Check sheet for the modelled part. Datum: model origin and axes. Units: mm. A direction names the side the tool comes from. Give positions to 0.01 mm unless a question says otherwise; leave off trailing zeros. Loops run counter-clockwise (first coordinate to the right, second up) from the corner with the lowest first, then second, coordinate; pieces in that order, holes last. Notation, with made-up numbers: (43, -21.75) - (76, -21.75) arc R14 cw to (76, 3.25) - close; hole circle Ø4 at (30, -25.5). An arc over 180 degrees is marked (long way). Answer in a Markdown table with one row per item. Add a question column.
(1) Thickness scan on L1, parallel to X at y = 1.35, z = -80; L2, parallel to X at y = 2.4, z = -32; L3, parallel to Z at x = -32, y = 3.55. Record the ranges inside material, lowest first.
(2) Set-up check for faces 5 (the face through (0, 2, -54)), 6 (the face through (10, 2, -47)): record each of +Z, -Z, +X, -X, +Y, -Y from which the full face is reachable in a straight line by a thin tool's end or side.
(3) Draft check along X on faces 1 (the face through (5.806, 1.972, -81.265)), 2 (the face through (2, 4, -31)), 3 (the face through (-3.01, 2.03, -2.85)), 4 (the face through (8, 2, 9)). Enter one of: released by +X, released by -X, zero draft, split by the parting line, or undercut.
(4) Sectioned sample at C-C on x = -21. Enter the section's corners in (y, z).
(5) Go/stop test with flat-tipped pins: P1, Ø4, axis at x = -31, z = 5, coming from the +Y side; P2, Ø1.5, axis at y = 3, z = -45.5, coming from the -X side; P3, Ø2, axis at x = -20.5, y = 2, coming from the -Z side. Record where each tip stops, or that it passes through.
(6) Sectioned sample at B-B on y = 3.25. Enter the section's corners in (x, z).
(7) Sectioned sample at A-A on x = -31.5. Enter the section's corners in (y, z).
(8) Sectioned sample at D-D on z = -64. Enter the section's corners in (x, y), then the cut area to 3 significant figures.
from build123d import *

# Parameters (mm, degrees)
SKETCH1_R           = 1.5
BOSS_EXTRUDE1_DEPTH = 4
SKETCH2_R           = 2.25
BOSS_EXTRUDE2_DEPTH = 4
FILLET1_R           = 10
FILLET2_R           = 5


with BuildPart() as part:
    # Sketch1 → Boss-Extrude1 (new body)
    with BuildSketch(Plane(origin=(0, 0, 0), x_dir=(1, 0, 0), z_dir=(0, 1, 0))):
        with BuildLine():
            Line((0, 0), (0, 100))
            ThreePointArc((0, 100), (5, 105), (10, 100))
            Line((10, 100), (10, 0))
            Line((10, 0), (0, 0))
        make_face()
        with Locations((5, 80)):
            Circle(SKETCH1_R, mode=Mode.SUBTRACT)
    extrude(amount=BOSS_EXTRUDE1_DEPTH)

    # Sketch2 → Boss-Extrude2 (add)
    with BuildSketch(Plane(origin=(0, 4, 0), x_dir=(1, 0, 0), z_dir=(0, 1, 0))):
        with BuildLine():
            Line((10, 0), (0, 0))
            Line((0, 0), (-45, 0))
            ThreePointArc((-45, 0), (-50, -5), (-45, -10))
            Line((-45, -10), (10, -10))
            Line((10, -10), (10, 0))
        make_face()
        with Locations((-45, -5)):
            Circle(SKETCH2_R, mode=Mode.SUBTRACT)
        with Locations((-31, -5)):
            Circle(SKETCH2_R, mode=Mode.SUBTRACT)
        with Locations((-9, -5)):
            Circle(SKETCH2_R, mode=Mode.SUBTRACT)
        with Locations((5, -5)):
            Circle(SKETCH2_R, mode=Mode.SUBTRACT)
    extrude(amount=-BOSS_EXTRUDE2_DEPTH)

    # Fillet1
    fillet1_edges = [part.edges().sort_by_distance(p)[0] for p in [
        (0, 2, 0),
    ]]
    fillet(fillet1_edges, radius=FILLET1_R)

    # Fillet2
    fillet2_edges = [part.edges().sort_by_distance(p)[0] for p in [
        (10, 2, 10),
    ]]
    fillet(fillet2_edges, radius=FILLET2_R)


solid = part.part
Reply:
| question | item | result |
|---|---|---|
| 1 | L1 | 0 to 3.5, 6.5 to 10 |
| 1 | L2 | 0 to 10 |
| 1 | L3 | 0 to 2.98, 7.02 to 10 |
| 2 | face 5 | -Z, -X, +Y, -Y |
| 2 | face 6 | +Z, -Z, +X, +Y, -Y |
| 3 | face 1 | undercut |
| 3 | face 2 | zero draft |
| 3 | face 3 | released by -X |
| 3 | face 4 | released by +X |
| 4 | outline | (0, 0) - (4, 0) - (4, 10) - (0, 10) - close |
| 5 | P1 | through |
| 5 | P2 | x = 0 |
| 5 | P3 | z = 0 |
| 6 | outline | (-45, 0) - (-10, 0) arc R10 cw to (0, -10) - (0, -100) arc R5 ccw to (10, -100) - (10, 5) arc R5 ccw to (5, 10) - (-45, 10) arc R5 ccw to start; hole circle Ø4.5 at (-45, 5); hole circle Ø4.5 at (-31, 5); hole circle Ø4.5 at (-9, 5); hole circle Ø4.5 at (5, 5); hole circle Ø3 at (5, -80) |
| 7 | outline | (0, 0) - (4, 0) - (4, 2.81) - (0, 2.81) - close; (0, 7.19) - (4, 7.19) - (4, 10) - (0, 10) - close |
| 8 | outline | (0, 0) - (10, 0) - (10, 4) - (0, 4) - close |
| 8 | area | 40.0 mm^2 |
